Build history of the part. All positions in model axes, mm. Give positions to 0.01 mm unless a question says otherwise; leave off trailing zeros. Loops run counter-clockwise (first coordinate to the right, second up) from the corner with the lowest first, then second, coordinate; pieces in that order, holes last. Notation, with made-up numbers: (66.25, -19.5) -> (121.25, -19.5) arc R7 cw to (121.25, -15.5) -> close; hole circle Ø9 at (-13, 30). An arc over 180 degrees is marked (long way). One line per question, with ' | ' between items. Start each with the question number.
(1) Slice it at B-B, the plane x = 430. Write the cut outline in (y, z), then the cut area to 3 significant figures.
(2) Flat gauge pin, fed straight in: pin 1 Ø4 at (x, z) = (377, -16) entering from +Y. Where does the tip first touch, or does it go through?
(3) Drill centre lines: L1, parallel to Z at x = 374.5, y = 6.75; L2, parallel to Y at x = 352.5, z = -17.25. Where is each one in solid material? Low to high. Write a range as from..to.
(4) Slice it at A-A, the plane y = 5.75. Write the cut outline in (x, z), then the cut area to 3 significant figures.
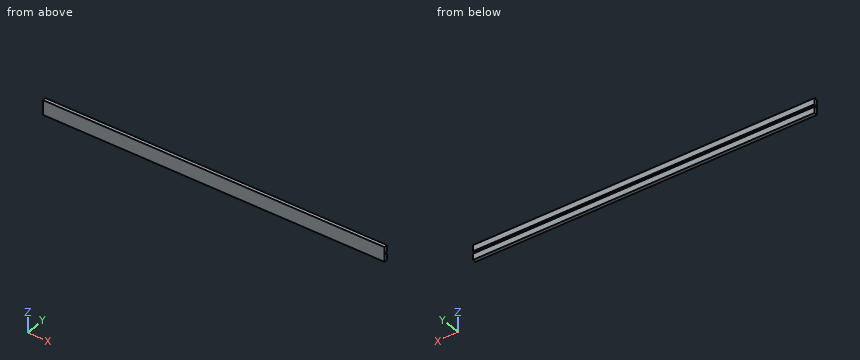
Autodesk Inventor part; units mm, degrees
ref_plane "YZ Plane" through (0, 0, 0) normal (1, 0, 0) x (0, 1, 0)
ref_plane "XZ Plane" through (0, 0, 0) normal (0, 1, 0) x (-1, 0, 0)
ref_plane "XY Plane" through (0, 0, 0) normal (0, 0, 1) x (1, 0, 0)
sketch "スケッチ1" plane through (0, 0, 0) normal (0, 1, 0) x (-1, 0, 0)
  line L0 (0, 0) -> (-700, 0)
  line L1 (-700, 0) -> (-700, -30)
  line L2 (-700, -30) -> (0, -30)
  line L3 (0, -30) -> (0, 0)
  dimension "d0" = 700
  dimension "d1" = 30
extrude "押し出し1" add sketch "スケッチ1" along normal blind 7
ref_plane "作業平面1" through (0, 7, 0) normal (0, 1, 0) x (1, 0, 0)
sketch "スケッチ2" plane through (0, 7, 0) normal (0, 1, 0) x (1, 0, 0)
  line L0 (0, 30) -> (0, 0)
  line L1 (0, 12.5) -> (700, 12.5)
  line L2 (700, 12.5) -> (700, 17.5)
  line L3 (700, 17.5) -> (0, 17.5)
  line L4 (0, 17.5) -> (0, 12.5)
  point P0 (0, 17.5)
  point P1 (0, 17.5)
  dimension "d5" = 5
  dimension "d6" = 700
  dimension "d7" = 5
extrude "押し出し2" cut sketch "スケッチ2" against normal blind 3
properties part number "guid"
Final values:
1) outline: (0, -30) -> (7, -30) -> (7, -17.5) -> (4, -17.5) -> (4, -12.5) -> (7, -12.5) -> (7, 0) -> (0, 0) -> close | area: 195 mm2
2) pin 1: y = 7
3) L1: -30..-17.5, -12.5..0 | L2: 0..4
4) outline: (0, -30) -> (700, -30) -> (700, -17.5) -> (0, -17.5) -> close; (0, -12.5) -> (700, -12.5) -> (700, 0) -> (0, 0) -> close | area: 17,500 mm2
